Geometry: final body of the model. Coordinates: model frame, mm. Face numbers are marked on the shaded views. Give positions to 0.01 mm unless a question says otherwise; leave off trailing zeros. Write each loop counter-clockwise with the first axis right and the second up, starting at its lowest first coordinate (ties: lowest second). Pieces come first, ordered by that corner, then holes. Notation, with made-up numbers: (-25.75, 26) - (3.25, 26) arc R16 cw to (3.25, 42) - close; hole circle Ø9 at (-34, 27). An arc over 180 degrees is marked (long way). Return JSON: item names as keys, results as strings.
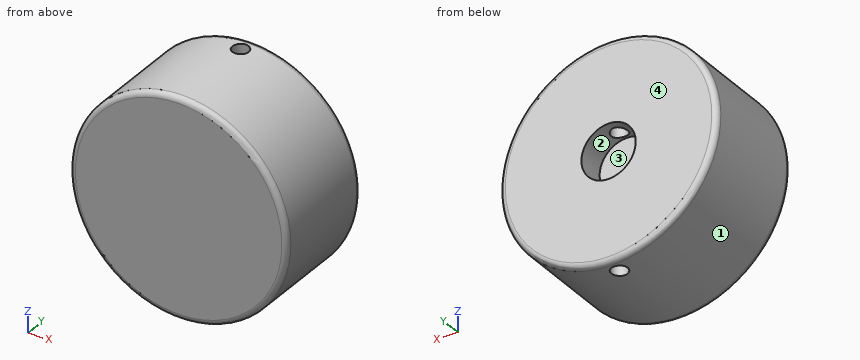
from build123d import *

# Parameters (mm, degrees)
SKETCH1_R           = 20
BOSS_EXTRUDE1_DEPTH = 20
SKETCH2_R           = 5
CUT_EXTRUDE1_DEPTH  = 5
SKETCH3_R           = 1.5
CUT_EXTRUDE2_DEPTH  = 49.989794856
FILLET1_R           = 1
FILLET2_R           = 1


with BuildPart() as part:
    # Sketch1 → Boss-Extrude1 (new body)
    with BuildSketch(Plane(origin=(0, 0, 0), x_dir=(1, 0, 0), z_dir=(0, 1, 0))):
        with Locations(Location((0, 0, 0), (0, 0, 270))):
            Circle(SKETCH1_R)
    extrude(amount=BOSS_EXTRUDE1_DEPTH)

    # Sketch2 → Cut-Extrude1 (cut)
    with BuildSketch(Plane(origin=(0, 20, 0), x_dir=(1, 0, 0), z_dir=(0, 1, 0))):
        with Locations(Location((0, 0, 0), (0, 0, 270))):
            Circle(SKETCH2_R)
    extrude(amount=-CUT_EXTRUDE1_DEPTH, mode=Mode.SUBTRACT)

    # Sketch3 → Cut-Extrude2 (cut, through all)
    with BuildSketch(Plane.XY.offset(20)):
        with Locations((0, 17)):
            Circle(SKETCH3_R)
    extrude(amount=-CUT_EXTRUDE2_DEPTH, mode=Mode.SUBTRACT)

    # Fillet1
    fillet1_edges = [part.edges().sort_by_distance(p)[0] for p in [
        (0, 0, -20),
    ]]
    fillet(fillet1_edges, radius=FILLET1_R)

    # Fillet2
    fillet2_edges = [part.edges().sort_by_distance(p)[0] for p in [
        (0, 20, -20),
    ]]
    fillet(fillet2_edges, radius=FILLET2_R)


solid = part.part
Q1. Pin query (flat end, axial travel): P1, Ø1, axis at x = -11.5, y = 7, coming from the +Z side; P2, Ø8, axis at x = -16, y = 6, coming from the +Z side; P3, Ø4, axis at y = 10.5, z = 9, coming from the -X side (3 decimals); P4, Ø1.8, axis at x = 0, y = 17, coming from the -Z side. Return the tip coordinate at first contact, or that it passes through.
Answer key:
{"P1": "stops at z = 16.7", "P2": "stops at z = 16", "P3": "stops at x = -18.735", "P4": "passes through"}
Q2. Mould query, pull axis X, two halves, no side actions, for the marked faces 1, 2, 3 and 4. Classes: pulls with the +X half, pulls with the -X half, needs draft (parallel to the pull), parting line crosses it, or undercut.
Answer key:
{"face 1": "parting line crosses it", "face 2": "undercut", "face 3": "undercut", "face 4": "needs draft"}
Q3. Section query C-C, the plane x = -1. Count the separate pieces of the cut face and the enclosed holes in it, plus the area to 3 significant figures.
Answer key:
{"separate pieces": "3", "enclosed holes": "0", "area": "682 mm^2"}
Q4. Section query D-D, the plane y = 8.5. Return the cut outline in (x, z), plus the area to 3 significant figures.
Answer key:
{"outline": "circle Ø40 at (0, 0)", "area": "1,260 mm^2"}
Q5. Section query A-A, the plane z = 0. Return the cut outline in (x, y).
Answer key:
{"outline": "(-20, 1) arc R1 ccw to (-19, 0) - (19, 0) arc R1 ccw to (20, 1) - (20, 19) arc R1 ccw to (19, 20) - (5, 20) - (5, 15) - (-5, 15) - (-5, 20) - (-19, 20) arc R1 ccw to (-20, 19) - close"}
Q6. Material intervals for probe 1 along X at (y, z) = (16, 0); probe 2 along Z at (x, y) = (-2, 16); probe 3 along Y at (x, z) = (-0.5, 1.5), sorted ascending. Write a range as [from, to].
Answer key:
{"probe 1": "x = [-20, -5], [5, 20]", "probe 2": "z = [-19.9, -4.58], [4.58, 19.9]", "probe 3": "y = [0, 15]"}
Q7. Section query B-B, the plane y = 17. Return the cut outline in (x, z).
Answer key:
{"outline": "(-1.5, -19.94) - (-1.5, -4.77) arc R5 cw to (-1.5, 4.77) - (-1.5, 19.94) arc R20 ccw to start; (1.5, -19.94) arc R20 ccw to (1.5, 19.94) - (1.5, 4.77) arc R5 cw to (1.5, -4.77) - close"}
